Verification items for the finished model (mm, model axes). A direction names the side the tool comes from. Give positions to 0.01 mm unless a question says otherwise; leave off trailing zeros. Loops run counter-clockwise (first coordinate to the right, second up) from the corner with the lowest first, then second, coordinate; pieces in that order, holes last. Notation, with made-up numbers: M -17,19.25 L 12,19.25 A24 cw 12,30.25 Z; hole C 64,-13 d10. An arc over 180 degrees is marked long. Write each question's results on one line, items separated by ' | '. Start each with the question number.
```python
from build123d import *

# Parameters (mm, degrees)
SKETCH1_W           = 118
SKETCH1_H           = 52
BOSS_EXTRUDE1_DEPTH = 2
CUT_EXTRUDE1_DEPTH  = 10
SKETCH4_W           = 38
SKETCH4_H           = 7
CUT_EXTRUDE2_DEPTH  = 10
SKETCH5_W           = 46.483490982
SKETCH5_H           = 11.25265215
CUT_EXTRUDE3_DEPTH  = 10
FILLET1_R           = 5
FILLET2_R           = 7
FILLET3_R           = 7
FILLET4_R           = 4
FILLET5_R           = 4


with BuildPart() as part:
    # Sketch1 → Boss-Extrude1 (new body)
    with BuildSketch(Plane.XY):
        Rectangle(SKETCH1_W, SKETCH1_H)
    extrude(amount=BOSS_EXTRUDE1_DEPTH)

    # Sketch3 → Cut-Extrude1 (cut)
    with BuildSketch(Plane.XY.offset(2)):
        with BuildLine():
            Line((-33.241745491, -23), (-33.241745491, -12))
            add(Edge.make_bspline(
                [(-33.241745491, -12), (-33.241745491, -6), (-45.86936562, -6)],
                knots=[3.141592654, 3.141592654, 3.141592654, 4.71238898, 4.71238898, 4.71238898], degree=2, weights=[1, 0.707106781, 1]))
            Line((-45.86936562, -6), (-59, -6))
            Line((-59, -6), (-59, -26))
            Line((-59, -26), (59, -26))
            Line((59, -26), (59, -6))
            Line((59, -6), (45.86936562, -6))
            add(Edge.make_bspline(
                [(45.86936562, -6), (33.241745491, -6), (33.241745491, -12)],
                knots=[1.570796327, 1.570796327, 1.570796327, 3.141592654, 3.141592654, 3.141592654], degree=2, weights=[1, 0.707106781, 1]))
            Line((33.241745491, -12), (33.241745491, -23))
            Line((33.241745491, -23), (-33.241745491, -23))
        make_face()
    extrude(amount=-CUT_EXTRUDE1_DEPTH, mode=Mode.SUBTRACT)

    # Sketch4 → Cut-Extrude2 (cut)
    with BuildSketch(Plane.XY.offset(2)):
        with Locations((0, 22.5)):
            Rectangle(SKETCH4_W, SKETCH4_H)
    extrude(amount=-CUT_EXTRUDE2_DEPTH, mode=Mode.SUBTRACT)

    # Sketch5 → Cut-Extrude3 (cut)
    with BuildSketch(Plane.XY.offset(2)):
        with Locations((0, -11.373673925)):
            Rectangle(SKETCH5_W, SKETCH5_H)
    extrude(amount=-CUT_EXTRUDE3_DEPTH, mode=Mode.SUBTRACT)

    # Fillet1
    fillet1_edges = [part.edges().sort_by_distance(p)[0] for p in [
        (-23.241745491, -17, 1),
        (-23.241745491, -5.74734785, 1),
        (23.241745491, -5.74734785, 1),
        (23.241745491, -17, 1),
    ]]
    fillet(fillet1_edges, radius=FILLET1_R)

    # Fillet2
    fillet2_edges = [part.edges().sort_by_distance(p)[0] for p in [
        (19, 19, 1),
        (-19, 19, 1),
    ]]
    fillet(fillet2_edges, radius=FILLET2_R - 0.0001)  # a hair under: the kernel refuses the full size

    # Fillet3
    fillet3_edges = [part.edges().sort_by_distance(p)[0] for p in [
        (19, 26, 1),
        (-19, 26, 1),
    ]]
    fillet(fillet3_edges, radius=FILLET3_R)

    # Fillet4
    fillet4_edges = [part.edges().sort_by_distance(p)[0] for p in [
        (59, -6, 1),
        (-59, -6, 1),
        (-33.241745491, -23, 1),
        (33.241745491, -23, 1),
    ]]
    fillet(fillet4_edges, radius=FILLET4_R)

    # Fillet5
    fillet5_edges = [part.edges().sort_by_distance(p)[0] for p in [
        (-59, 26, 1),
        (59, 26, 1),
    ]]
    fillet(fillet5_edges, radius=FILLET5_R)


solid = part.part
```
1. Section check A-A, the plane x = 1. Record the boundary of the cut face in (y, z).
2. Depth check by flat-ended pin: pin 1 Ø1 at (x, z) = (-49, 0.5) entering from -Y; pin 2 Ø1 at (y, z) = (-15, 1.5) entering from +X; pin 3 Ø4 at (x, y) = (20, 21) entering from -Z; pin 4 Ø1 at (y, z) = (-16, 1.5) entering from -X. Enter the tip coordinate at first touch or a pass-through.
3. Thickness scan on probe 1 along Y at (x, z) = (-6.5, 0.2); probe 2 along Y at (x, z) = (-51.5, 1.6); probe 3 along X at (y, z) = (-13, 1.15). Record the ranges inside material, lowest first.
4. Release check for a two-part mould opening along X. For faces 1 (the face through (15.456, 19.912, 0.986)), 2 (the face through (57.797, 24.859, 1.014)), 3 (the face through (-21.74, -15.57, 0.99)), 4 (the face through (-57.859, -4.797, 0.986)) record: released by +X, released by -X, zero draft, split by the parting line, or undercut.
5. Set-up check for faces 5 (the face through (0, 19, 1)), 6 (the face through (-50, -6, 1)), 7 (the face through (32.04, -21.86, 0.99)), 8 (the face through (0, -17, 1)): record each of +Z, -Z, +X, -X, +Y, -Y from which the full face is reachable in a straight line by a thin tool's end or side.
Filled sheet:
1) outline: M -23,0 L -17,0 L -17,2 L -23,2 Z; M -5.75,0 L 19,0 L 19,2 L -5.75,2 Z
2) pin 1: y = -6 | pin 2: x = 33.24 | pin 3: z = 0 | pin 4: x = -33.24
3) probe 1: -23 to -17, -5.75 to 19 | probe 2: -6 to 26 | probe 3: -33.24 to -23.14, 23.14 to 33.24
4) face 1: undercut | face 2: released by +X | face 3: undercut | face 4: released by -X
5) face 5: +Z, -Z, +Y | face 6: +Z, -Z, -X, -Y | face 7: +Z, -Z, +X, -Y | face 8: +Z, -Z
